```python
from build123d import *

# Parameters (mm, degrees)
SKETCH_R     = 7
PAD_DEPTH    = 4
SKETCH001_R  = 3.925
PAD001_DEPTH = 19
CHAMFER_SIZE = 1
FILLET_R     = 1


with BuildPart() as part:
    # Sketch → Pad (new body)
    with BuildSketch(Plane.XY):
        Circle(SKETCH_R)
    extrude(amount=PAD_DEPTH)

    # Sketch001 (on Face3 of Pad) → Pad001 (join)
    with BuildSketch(Plane.XY.offset(4)):
        Circle(SKETCH001_R)
    extrude(amount=PAD001_DEPTH)

    # Chamfer
    chamfer_edges = [part.edges().sort_by_distance(p)[0] for p in [
        (-3.925, 0, 23),
    ]]
    chamfer(chamfer_edges, length=CHAMFER_SIZE)

    # Fillet
    fillet_edges = [part.edges().sort_by_distance(p)[0] for p in [
        (-7, 0, 0),
    ]]
    fillet(fillet_edges, radius=FILLET_R)


solid = part.part
```
Part model, mm, in its own coordinate system. A direction names the side the tool comes from. Round coordinates to 2 decimals unless told otherwise and drop trailing zeros. Order: outer loops, then holes, each group sorted by start corner. A loop starts at its lowest first (then second) coordinate and runs counter-clockwise, first axis right, second up. Notation, with made-up numbers: M 71,60 L 110,60 A17 cw 110,88 Z; hole C 24.5,-26.75 d3. An arc over 180 degrees is marked long. Answer in a Markdown table with one row per item. Add a question column.
Q1. Cut at A-A on x = 0. Give the cut face in (y, z) (3 decimals), and give its area (3 significant figures).
Q2. Cut at D-D on z = 10.5. Give the cut face in (x, y) (3 decimals), and give its area (3 significant figures).
Q3. Wall check: L1, parallel to Y at x = 0, z = 9 (3 decimals); L2, parallel to Z at x = -4.25, y = 3; L3, parallel to X at y = 0.75, z = 1.25. Give the ranges that are in metal, low to high. Write a range as from..to.
Q4. Cut at C-C on z = 2.75. Give the cut face in (x, y), and give its area (3 significant figures).
Q5. 3-axis set-ups, long thin cutter, end or side, ignore diameter. For faces 1 (the face through (3, -3, 4)), 2 (the face through (0, 0, 23)): which of +Z, -Z, +X, -X, +Y, -Y reach the whole face in a straight line?
Q6. Mould opens along X. For faces 3 (the face through (6.466, -2.681, 2.479)), 4 (the face through (0, 0, 0)) say: +X half, -X half, draft (parallel to the pull), parting line (faces both ways), or undercut.
Established:
| question | item | result |
|---|---|---|
| 1 | outline | M -7,1 A1 ccw -6,0 L 6,0 A1 ccw 7,1 L 7,4 L 3.925,4 L 3.925,22 L 2.925,23 L -2.925,23 L -3.925,22 L -3.925,4 L -7,4 Z |
| 1 | area | 204 mm2 |
| 2 | outline | C 0,0 d7.85 |
| 2 | area | 48.4 mm2 |
| 3 | L1 | y = -3.925..3.925 |
| 3 | L2 | z = 0..4 |
| 3 | L3 | x = -6.96..6.96 |
| 4 | outline | C 0,0 d14 |
| 4 | area | 154 mm2 |
| 5 | face 1 | +Z |
| 5 | face 2 | +Z, +X, -X, +Y, -Y |
| 6 | face 3 | parting line |
| 6 | face 4 | draft |
